Check sheet for the modelled part. Datum: model origin and axes. Units: mm. A direction names the side the tool comes from. Round coordinates to 2 decimals unless told otherwise and drop trailing zeros. Write each loop counter-clockwise with the first axis right and the second up, starting at its lowest first coordinate (ties: lowest second). Pieces come first, ordered by that corner, then holes. Notation, with made-up numbers: (78.25, 88.25) - (90.25, 88.25) arc R17 ccw to (90.25, 107.25) - close; hole circle Ø1 at (77.25, -16). An arc over 180 degrees is marked (long way). Use one line per item in the form item = value. Start each with the question number.
1) Scan lines: probe 1 along Z at (x, y) = (-1, -9.5); probe 2 along Z at (x, y) = (-8.5, -7); probe 3 along X at (y, z) = (8.5, 2.25). Record each from-to range of solid material in increasing order.
2) Set-up check for faces 1 (the face through (-0.634, -2.855, 6.226)), 2 (the face through (0, -4, 0)): record each of +Z, -Z, +X, -X, +Y, -Y from which the full face is reachable in a straight line by a thin tool's end or side.
3) Section check B-B (y = 0). Record the boundary of the cut face in (x, z) (3 decimals), then the cut area to 3 significant figures.
4) Section check A-A (x = 0). Record the boundary of the cut face in (y, z) (3 decimals).
5) Section check C-C (z = 6.5). Record the boundary of the cut face in (x, y) (3 decimals), then the cut area to 3 significant figures.
6) Section check D-D (x = 8). Record the boundary of the cut face in (y, z), then the cut area to 3 significant figures.
7) Gauge pin test, flat ends, axial feed: P1, Ø1, axis at x = -4, z = 2, coming from the +Y side; P2, Ø3, axis at x = 13.5, y = -14.5, coming from the -Z side; P3, Ø10, axis at x = -11, y = 1.5, coming from the +Z side; P4, Ø1.5, axis at x = -3, z = 5, coming from the +Y side. Record the tip position at first contact, or that the pin passes through.
from build123d import *

# Parameters (mm, degrees)
F0_R     = 20
F1_DEPTH = 1
F2_R     = 9.925
F3_DEPTH = 3.5
F4_R     = 2.925
F5_DEPTH = 3.5
F6_W     = 16
F6_H     = 9
F7_DEPTH = 25


with BuildPart() as f1:
    # F0 (on Top) → F1 (new body)
    with BuildSketch(Plane.XY):
        Circle(F0_R)
    extrude(amount=F1_DEPTH)

    # F2 (on face) → F3 (join)
    with BuildSketch(Plane.XY.offset(1)):
        Circle(F2_R)
    extrude(amount=F3_DEPTH)

    # F4 (on face) → F5 (join)
    with BuildSketch(Plane.XY.offset(4.5)):
        Circle(F4_R)
    extrude(amount=F5_DEPTH)

    # F6 (on face) → F7 (cut)
    with BuildSketch(Plane.XY.offset(1)):
        with Locations((8, 16.5)):
            Rectangle(F6_W, F6_H)
        with Locations((-8, 16.5)):
            Rectangle(F6_W, F6_H)
    extrude(amount=-F7_DEPTH, mode=Mode.SUBTRACT)


solid = f1.part
Results are:
q1.probe_1 = 0 to 4.5
q1.probe_2 = 0 to 1
q1.probe_3 = -5.12 to 5.12
q2.face_1 = +Z
q2.face_2 = -Z, +X, -X, +Y, -Y
q3.outline = (-20, 0) - (20, 0) - (20, 1) - (9.925, 1) - (9.925, 4.5) - (2.925, 4.5) - (2.925, 8) - (-2.925, 8) - (-2.925, 4.5) - (-9.925, 4.5) - (-9.925, 1) - (-20, 1) - close
q3.area = 130 mm²
q4.outline = (-20, 0) - (12, 0) - (12, 1) - (9.925, 1) - (9.925, 4.5) - (2.925, 4.5) - (2.925, 8) - (-2.925, 8) - (-2.925, 4.5) - (-9.925, 4.5) - (-9.925, 1) - (-20, 1) - close
q5.outline = circle Ø5.85 at (0, 0)
q5.area = 26.9 mm²
q6.outline = (-18.33, 0) - (12, 0) - (12, 1) - (5.87, 1) - (5.87, 4.5) - (-5.87, 4.5) - (-5.87, 1) - (-18.33, 1) - close
q6.area = 71.4 mm²
q7.P1 = 9.29
q7.P2 = 0
q7.P3 = 4.5
q7.P4 = 9.62
